Here's how the part is built. I have some questions about the finished solid (model axes, mm). A direction names the side the tool comes from. Round coordinates to 2 decimals unless told otherwise and drop trailing zeros. Write each loop counter-clockwise with the first axis right and the second up, starting at its lowest first coordinate (ties: lowest second). Pieces come first, ordered by that corner, then holes. Notation, with made-up numbers: (-5.75, 6) -> (2.25, 6) arc R27 ccw to (2.25, 26) -> close; hole circle Ø1 at (42, -13). An arc over 180 degrees is marked (long way). Answer as CSV lines item,"result".
from build123d import *

# Parameters (mm, degrees)
SKETCH1_R           = 50
BOSS_EXTRUDE1_DEPTH = 20
SKETCH2_R           = 47
BOSS_EXTRUDE2_DEPTH = 23
SKETCH3_R           = 3
SKETCH3_R_2         = 10
CUT_EXTRUDE1_DEPTH  = 83.758685345
SKETCH5_R           = 2.5
CUT_EXTRUDE3_DEPTH  = 25
CIRPATTERN1_COUNT   = 4


with BuildPart() as part:
    # Sketch1 → Boss-Extrude1 (new body)
    with BuildSketch(Plane.XY):
        Circle(SKETCH1_R)
    extrude(amount=BOSS_EXTRUDE1_DEPTH)

    # Sketch2 → Boss-Extrude2 (add)
    with BuildSketch(Plane.XY.offset(20)):
        Circle(SKETCH2_R)
    extrude(amount=BOSS_EXTRUDE2_DEPTH)

    # Sketch3 → Cut-Extrude1 (cut, through all)
    with BuildSketch(Plane.XY.offset(43)):
        with Locations((0, 40)):
            Circle(SKETCH3_R)
        with Locations((34.641016151, -20)):
            Circle(SKETCH3_R)
        with Locations((-34.641016151, -20)):
            Circle(SKETCH3_R)
        with Locations((0, -25)):
            Circle(SKETCH3_R)
        with Locations((0, 25)):
            Circle(SKETCH3_R)
        Circle(SKETCH3_R_2)
    extrude(amount=-CUT_EXTRUDE1_DEPTH, mode=Mode.SUBTRACT)

    # Sketch5 → Cut-Extrude3 (cut)
    with BuildSketch(Plane.ZY.offset(-50)):
        with Locations((33, 0)):
            Circle(SKETCH5_R)
    cut_extrude3 = extrude(amount=CUT_EXTRUDE3_DEPTH, mode=Mode.SUBTRACT)

    # CirPattern1: Cut-Extrude3 ×4 about axis
    cirpattern1_axis = Axis((0, 0, 43), (0, 0, -1))
    for i in range(1, CIRPATTERN1_COUNT):
        add(cut_extrude3.rotate(cirpattern1_axis, i * 360 / CIRPATTERN1_COUNT), mode=Mode.SUBTRACT)


solid = part.part
Item 1: If we mould it in two halves opening along Z, with no side actions, what happens to faces 1 (the cylindrical face through (0, -22, 22)), 2 (the flat face through (-25, 0, 33)), 3 (the flat face through (-1, 11, 43))? For each: pulls with the +Z half, pulls with the -Z half, needs draft (parallel to the pull), parting line crosses it, or undercut.
Results found:
face 1,"needs draft"
face 2,"undercut"
face 3,"pulls with the +Z half"
Item 2: Suppose I cut it at D-D, the plane x = 0. State how many separate pieces and enclosed holes the cut face has, then the cut area to 3 significant figures.
Results found:
separate pieces,"8"
enclosed holes,"0"
area,"2,370 mm²"
Item 3: For faces 4 (the flat face through (-34, -33, 20)), 5 (the flat face through (25, 0, 33)), 6 (the cylindrical face through (-0.96, -36.97, 35.31)), 7 (the cylindrical face through (-36.15, 2.22, 34.15)), 8 (the cylindrical face through (-0.1, 45, 30.5)), which set-ups out of +Z, -Z, +X, -X, +Y, -Y let a thin tool reach every point of the face, with its end or its side?
Results found:
face 4,"+Z"
face 5,"+X"
face 6,"-Y"
face 7,"-X"
face 8,"+Y"
Item 4: Will these pins go through, and if not, where does the flat tip stop? pin 1 (1.5 mm diameter, centred on x = -26.5, z = 10, fed in from +Y); pin 2 (5 mm diameter, centred on x = 5, z = 35.5, fed in from -Y); pin 3 (10 mm diameter, centred on y = 28, z = 30, fed in from +X).
Results found:
pin 1,"stops at y = 42.86"
pin 2,"stops at y = -46.93"
pin 3,"stops at x = 40.99"
Item 5: Suppose I cut it at B-B, the plane z = 38. List the corners of the cut face in (x, y) for me.
Results found:
outline,"circle Ø94 at (0, 0); hole circle Ø6 at (-34.64, -20); hole circle Ø20 at (0, 0); hole circle Ø6 at (0, -25); hole circle Ø6 at (0, 25); hole circle Ø6 at (0, 40); hole circle Ø6 at (34.64, -20)"
Item 6: Suppose I cut it at C-C, the plane y = -20. List the corners of the cut face in (x, z) for me.
Results found:
outline,"(-45.83, 0) -> (-37.64, 0) -> (-37.64, 43) -> (-42.53, 43) -> (-42.53, 20) -> (-45.83, 20) -> close; (-31.64, 0) -> (31.64, 0) -> (31.64, 43) -> (-31.64, 43) -> close; (37.64, 0) -> (45.83, 0) -> (45.83, 20) -> (42.53, 20) -> (42.53, 43) -> (37.64, 43) -> close"
Item 7: Suppose I cut it at A-A, the plane y = 0. List the corners of the cut face in (x, z) for me.
Results found:
outline,"(-50, 0) -> (-10, 0) -> (-10, 43) -> (-47, 43) -> (-47, 35.5) -> (-25, 35.5) -> (-25, 30.5) -> (-47, 30.5) -> (-47, 20) -> (-50, 20) -> close; (10, 0) -> (50, 0) -> (50, 20) -> (47, 20) -> (47, 30.5) -> (25, 30.5) -> (25, 35.5) -> (47, 35.5) -> (47, 43) -> (10, 43) -> close"
Item 8: I need wall thicknesses on L1, parallel to Y at x = 0, z = 10; L2, parallel to Y at x = 0, z = 22; L3, parallel to Z at x = 31, y = 0. Which ranges of each line are inside material? Lowest first, please.
Results found:
L1,"y = -50 to -28, -22 to -10, 10 to 22, 28 to 37, 43 to 50"
L2,"y = -47 to -28, -22 to -10, 10 to 22, 28 to 37, 43 to 47"
L3,"z = 0 to 30.5, 35.5 to 43"
